Design review of the part shown in the three views and the two pictorial views. Dimensions are in mm from the part's minimum x, y and z. Coordinates: 2 decimals unless noted, no trailing zeros. Loops run counter-clockwise (first coordinate to the right, second up) from the corner with the lowest first, then second, coordinate; pieces in that order, holes last.
Q1. Add section C-C on z = 295. Give the boundary of the cut face in (x, y).
Q2. Add section B-B on y = 460. Give the boundary of the cut face in (x, z), and give its area (3 significant figures).
Q3. Wall thickness on probe 1 along Y at (x, z) = (35, 939); probe 2 along Z at (x, y) = (34, 226.5) (1 decimal); probe 3 along Y at (x, z) = (12.5, 146.5): over which ranges is each line inside the solid? List them lowest first.
Q4. For P1, Ø4, axis at x = 13.5, z = 474, coming from the +Y side; P2, Ø4, axis at x = 8, y = 365, coming from the -Z side (1 decimal); P3, Ø1.5, axis at x = 30, y = 387.5, coming from the +Z side, all flat-tipped, find the tip position at first contact; note any pin that passes through.
Q5. Add section A-A on x = 18. Give the boundary of the cut face in (y, z), and give its area (3 significant figures).
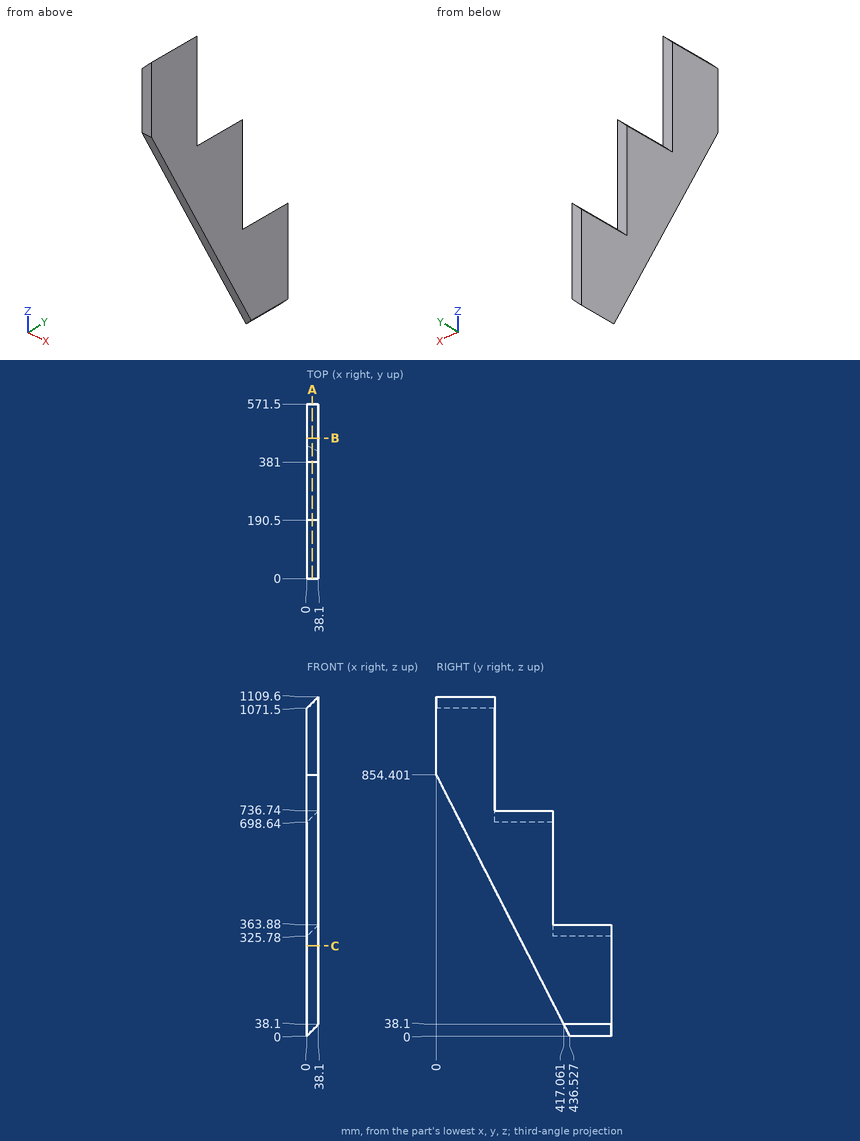
Entries:
1. outline: (0, 285.81) - (38.1, 285.81) - (38.1, 571.5) - (0, 571.5) - close
2. outline: (0, 0) - (38.1, 38.1) - (38.1, 363.88) - (0, 325.78) - close
2. area: 12,400 mm2
3. probe 1: y = 0 to 190.5
3. probe 2: z = 411.1 to 732.6
3. probe 3: y = 361.68 to 571.5
4. P1: stops at y = 381
4. P2: stops at z = 136.1
4. P3: stops at z = 356.53
5. outline: (0, 854.4) - (427.33, 18) - (571.5, 18) - (571.5, 343.78) - (381, 343.78) - (381, 716.64) - (190.5, 716.64) - (190.5, 1089.5) - (0, 1089.5) - close
5. area: 221,000 mm2
